from build123d import *

# Parameters (mm, degrees)
SKETCH1_R                   = 28.5
SKETCH1_R_2                 = 21
BOSS_EXTRUDE1_DEPTH         = 11
BOSS_EXTRUDE2_START         = -35.5
SKETCH1_3_R                 = 40
SKETCH1_3_R_2               = 28.5
SKETCH1_3_R_3               = 21
BOSS_EXTRUDE2_DEPTH         = 35.5
M3_TAPPED_HOLE1_D           = 2.5
M3_TAPPED_HOLE1_DEPTH       = 5
M3_TAPPED_HOLE1_CSINK_D     = 3.05
M3_TAPPED_HOLE1_CSINK_ANGLE = 90
M3_TAPPED_HOLE1_TIP         = 0.751075774
BOSS_EXTRUDE3_START         = 15.5
SKETCH5_R                   = 31
SKETCH5_R_2                 = 21
BOSS_EXTRUDE3_DEPTH         = 15.5


with BuildPart() as part:
    # Sketch1 → Boss-Extrude1 (new body)
    # profile 1 of 2: a face of its own
    with BuildSketch(Plane.XY):
        Circle(SKETCH1_R)
        Circle(SKETCH1_R_2, mode=Mode.SUBTRACT)
    # profile 2 of 2: a face of its own
    with BuildSketch(Plane.XY):
        Circle(SKETCH1_R_2)
    extrude(amount=BOSS_EXTRUDE1_DEPTH)

    # Sketch1_3 → Boss-Extrude2 (add)
    # profile 1 of 2: a face of its own
    with BuildSketch(Plane.XY.offset(BOSS_EXTRUDE2_START)):
        Circle(SKETCH1_3_R)
        Circle(SKETCH1_3_R_2, mode=Mode.SUBTRACT)
    # profile 2 of 2: a face of its own
    with BuildSketch(Plane.XY.offset(BOSS_EXTRUDE2_START)):
        Circle(SKETCH1_3_R_2)
        Circle(SKETCH1_3_R_3, mode=Mode.SUBTRACT)
    extrude(amount=BOSS_EXTRUDE2_DEPTH)

    # M3 Tapped Hole1
    with Locations(Plane(origin=(0, 0, -35.5), x_dir=(-1, 0, 0), z_dir=(0, 0, -1))):
        with Locations((0, 37), (26.162950904, 26.162950904), (37, 0), (26.162950904, -26.162950904), (0, -37), (-26.162950904, -26.162950904), (-37, 0), (-26.162950904, 26.162950904)):
            CounterSinkHole(M3_TAPPED_HOLE1_D / 2, M3_TAPPED_HOLE1_CSINK_D / 2, depth=M3_TAPPED_HOLE1_DEPTH, counter_sink_angle=M3_TAPPED_HOLE1_CSINK_ANGLE)
            with Locations((0, 0, -(M3_TAPPED_HOLE1_DEPTH + M3_TAPPED_HOLE1_TIP / 2))):  # 118° drill point
                Cone(0, M3_TAPPED_HOLE1_D / 2, M3_TAPPED_HOLE1_TIP, mode=Mode.SUBTRACT)

    # Sketch5 → Boss-Extrude3 (add)
    with BuildSketch(Plane(origin=(0, 0, -35.5), x_dir=(-1, 0, 0), z_dir=(0, 0, -1)).offset(BOSS_EXTRUDE3_START)):
        with Locations(Location((0, 0, 0), (0, 0, 180))):
            Circle(SKETCH5_R)
        with Locations(Location((0, 0, 0), (0, 0, 180))):
            Circle(SKETCH5_R_2, mode=Mode.SUBTRACT)
    extrude(amount=-BOSS_EXTRUDE3_DEPTH)


solid = part.part
Geometry: final body of the model. Coordinates: model frame, mm. A direction names the side the tool comes from. Coordinates: 2 decimals unless noted, no trailing zeros. Loops run counter-clockwise (first coordinate to the right, second up) from the corner with the lowest first, then second, coordinate; pieces in that order, holes last. Notation, with made-up numbers: (54, 9.5) - (80, 9.5) arc R37 cw to (80, 45.5) - close; hole circle Ø4 at (-19, 79.25). An arc over 180 degrees is marked (long way). Put each result on its own line as item: value. Start each with the question number.
Q1. Pull-direction query (X, two-part tool) for faces 3 (the cylindrical face through (26.327, -10.916, 5.423)), 4 (the flat face through (-9.4, 27.2, 0)), 5 (the conical face through (-26.116, -26.375, -29.879)); classes: released by +X, released by -X, zero draft, split by the parting line, or undercut.
Q2. Cut plane A-A, the plane z = -16. Return loops of the section in (x, y).
Q3. Cut plane C-C, the plane z = 5. Return loops of the section in (x, y), and give its area (3 significant figures).
Q4. Cut plane B-B, the plane x = 19.5. Return loops of the section in (y, z), and give its area (3 significant figures).
Q5. Pin query (flat end, axial travel): pin 1 Ø4 at (x, y) = (-37, 0) entering from +Z; pin 2 Ø12 at (x, z) = (-24, 1.5) entering from +Y; pin 3 Ø10 at (y, z) = (-9.5, -18) entering from +X. Return the tip coordinate at first contact, or that it passes through.
Q6. Set-up query: faces 1 (the cylindrical face through (25.892, 24.943, -32.829)), 2 (the flat face through (6.5, 20.2, -51)). Return all of +Z, -Z, +X, -X, +Y, -Y with unobstructed straight access to the full face (end or side cutting, diameter ignored); none if empty.
Q7. Line query: line 1 (Y direction, x = 0, z = -32.35); line 2 (Z direction, x = 12, y = 16.5); line 3 (Y direction, x = -1.5, z = -0.5). Output: solid intervals per line, ascending.
Q8. Cut plane D-D, the plane x = -15. Return loops of the section in (y, z), and give its area (3 significant figures).
Filled sheet:
1. face 3: split by the parting line
1. face 4: zero draft
1. face 5: undercut
2. outline: circle Ø80 at (0, 0); hole circle Ø42 at (0, 0)
3. outline: circle Ø57 at (0, 0)
3. area: 2,550 mm²
4. outline: (-34.92, -35.5) - (-24.1, -35.5) - (-24.1, -51) - (-7.79, -51) - (-7.79, 0) - (7.79, 0) - (7.79, -51) - (24.1, -51) - (24.1, -35.5) - (34.92, -35.5) - (34.92, 0) - (20.78, 0) - (20.78, 11) - (-20.78, 11) - (-20.78, 0) - (-34.92, 0) - close
4. area: 2,890 mm²
5. pin 1: z = 0
5. pin 2: y = 35.62
5. pin 3: x = 39.75
6. face 1: -Z
6. face 2: -Z, +X, -X, +Y, -Y
7. line 1: -40 to -38.25, -35.75 to -21, 21 to 35.75, 38.25 to 40
7. line 2: 0 to 11
7. line 3: -39.97 to -20.95, 20.95 to 39.97
8. outline: (-37.08, -35.5) - (-27.13, -35.5) - (-27.13, -51) - (-14.7, -51) - (-14.7, 0) - (14.7, 0) - (14.7, -51) - (27.13, -51) - (27.13, -35.5) - (37.08, -35.5) - (37.08, 0) - (24.23, 0) - (24.23, 11) - (-24.23, 11) - (-24.23, 0) - (-37.08, 0) - close
8. area: 2,510 mm²
